```python
from build123d import *

# Parameters (mm, degrees)
SKETCH41_W                                    = 104.14
SKETCH41_H                                    = 148.59
SKETCH41_R                                    = 9.525
EXTRUDE16_DEPTH                               = 16.51
SKETCH42_W                                    = 19.05
SKETCH42_H                                    = 19.05
SKETCH42_W_2                                  = 13.97
SKETCH42_W_3                                  = 12.7
SKETCH42_H_2                                  = 15.24
EXTRUDE17_DEPTH                               = 2.54
F_1_4_CLEARANCE_HOLE3_AT_2_COUNT              = 2
F_1_4_CLEARANCE_HOLE3_AT_2_PITCH              = 88.9
F_1_4_CLEARANCE_HOLE3_AT_3_COUNT              = 2
F_1_4_CLEARANCE_HOLE3_AT_3_PITCH              = 49.6966108
PRESS_PIN_HOLES_FOR_MAGNET_BRACKET_P_2_COUNT  = 2
PRESS_PIN_HOLES_FOR_MAGNET_BRACKET_P_2_PITCH  = 88.9
F_3_32_0_09375_DIAMETER_HOLE1_D               = 2.38125
CBORE_FOR_1_4_SOCKET_HEAD_CAP_SCREW1_AT_COUNT = 2
CBORE_FOR_1_4_SOCKET_HEAD_CAP_SCREW1_AT_PITCH = 57.15
F_1_8_0_125_DIAMETER_HOLE1_AT_2_COUNT         = 2
F_1_8_0_125_DIAMETER_HOLE1_AT_2_PITCH         = 69.85
TAPPED_HOLE_FOR_8_32_HELICOIL1_AT_2_COUNT     = 2
TAPPED_HOLE_FOR_8_32_HELICOIL1_AT_2_PITCH     = 83.29041666
CHAMFER1_SIZE                                 = 5.08


with BuildPart() as part:
    # Sketch41 → Extrude16 (new body)
    with BuildSketch(Plane(origin=(0, 0, 0), x_dir=(1, 0, 0), z_dir=(0, 1, 0))):
        with Locations((0, -36.195)):
            Rectangle(SKETCH41_W, SKETCH41_H)
        with Locations(Location((0, -44.45, 0), (0, 0, 270))):  # turned: the seam where the file's is
            Circle(SKETCH41_R, mode=Mode.SUBTRACT)
    extrude(amount=EXTRUDE16_DEPTH)

    # Sketch42 → Extrude17 (add)
    with BuildSketch(Plane.XZ):
        with Locations((-28.575, 100.965)):
            Rectangle(SKETCH42_W, SKETCH42_H)
        with Locations((45.085, -10.795)):
            Rectangle(SKETCH42_W_2, SKETCH42_H)
        with Locations((0, -30.48)):
            Rectangle(SKETCH42_W_3, SKETCH42_H_2)
        with Locations((-45.085, -10.795)):
            Rectangle(SKETCH42_W_2, SKETCH42_H)
        with Locations((28.575, 100.965)):
            Rectangle(SKETCH42_W, SKETCH42_H)
    extrude(amount=EXTRUDE17_DEPTH)

    # Sketch43 → 1/4 Clearance Hole3 (revolve, cut)
    with BuildSketch(Plane(origin=(-44.45, -2.54, -8.255), x_dir=(0, 0, -1), z_dir=(1, 0, 0))):
        Polygon((0, 0), (0, 19.05), (3.9624, 19.05), (3.57124, 18.65884), (3.57124, 0.39116), (3.9624, 0), align=None)
    f_1_4_clearance_hole3 = revolve(axis=Axis((-44.45, -8.89, -8.255), (0, 1, 0)), mode=Mode.SUBTRACT)

    # 1/4 Clearance Hole3 at 2: 1/4 Clearance Hole3 ×2
    with Locations(*[(i * F_1_4_CLEARANCE_HOLE3_AT_2_PITCH, 0, 0) for i in range(1, F_1_4_CLEARANCE_HOLE3_AT_2_COUNT)]):
        add(f_1_4_clearance_hole3, mode=Mode.SUBTRACT)

    # 1/4 Clearance Hole3 at 3: 1/4 Clearance Hole3 ×2
    with Locations(*[Vector(0.894427191, 0, -0.447213595) * (i * F_1_4_CLEARANCE_HOLE3_AT_3_PITCH) for i in range(1, F_1_4_CLEARANCE_HOLE3_AT_3_COUNT)]):
        add(f_1_4_clearance_hole3, mode=Mode.SUBTRACT)

    # Sketch39 → Press Pin holes for Magnet Bracket Pins (revolve, cut)
    with BuildSketch(Plane(origin=(-44.45, -2.54, -16.51), x_dir=(0, 0, -1), z_dir=(1, 0, 0))):
        Polygon((0, 0), (0, 7.303866233), (1.5875, 6.35), (1.5875, 1.524), (1.6002, 1.524), (1.6002, 0.3048), (1.905, 0), align=None)
    press_pin_holes_for_magnet_bracket_pins = revolve(axis=Axis((-44.45, -8.89, -16.51), (0, 1, 0)), mode=Mode.SUBTRACT)

    # Press Pin holes for Magnet Bracket P 2: Press Pin holes for Magnet Bracket Pins ×2
    with Locations(*[(i * PRESS_PIN_HOLES_FOR_MAGNET_BRACKET_P_2_PITCH, 0, 0) for i in range(1, PRESS_PIN_HOLES_FOR_MAGNET_BRACKET_P_2_COUNT)]):
        add(press_pin_holes_for_magnet_bracket_pins, mode=Mode.SUBTRACT)

    # 3/32 (0.09375) Diameter Hole1 (through all)
    with Locations(Plane(origin=(0, 16.51, 0), x_dir=(-1, 0, 0), z_dir=(0, 1, 0))):
        with Locations((44.45, -16.51), (-44.45, -16.51)):
            Hole(F_3_32_0_09375_DIAMETER_HOLE1_D / 2)

    # Sketch7 → CBORE for 1/4 Socket Head Cap Screw1 (revolve, cut)
    with BuildSketch(Plane(origin=(-28.575, 16.51, 97.79), x_dir=(0, 0, 1), z_dir=(1, 0, 0))):
        Polygon((0, 0), (0, 19.050025), (3.9624, 19.050025), (3.57124, 18.658865), (3.57124, 6.35), (5.55625, 6.35), (5.55625, 0), align=None)
    cbore_for_1_4_socket_head_cap_screw1 = revolve(axis=Axis((-28.575, 22.86, 97.79), (0, -1, 0)), mode=Mode.SUBTRACT)

    # CBORE for 1/4 Socket Head Cap Screw1 at: CBORE for 1/4 Socket Head Cap Screw1 ×2
    with Locations(*[(i * CBORE_FOR_1_4_SOCKET_HEAD_CAP_SCREW1_AT_PITCH, 0, 0) for i in range(1, CBORE_FOR_1_4_SOCKET_HEAD_CAP_SCREW1_AT_COUNT)]):
        add(cbore_for_1_4_socket_head_cap_screw1, mode=Mode.SUBTRACT)

    # Sketch45 → 1/8 (0.125) Diameter Hole1 (revolve, cut)
    with BuildSketch(Plane(origin=(-34.925, -2.54, 105.41), x_dir=(0, 0, -1), z_dir=(1, 0, 0))):
        Polygon((0, 0), (0, 19.05), (1.905, 19.05), (1.63195, 18.77695), (1.63195, 0.27305), (1.905, 0), align=None)
    f_1_8_0_125_diameter_hole1 = revolve(axis=Axis((-34.925, -8.89, 105.41), (0, 1, 0)), mode=Mode.SUBTRACT)

    # 1/8 (0.125) Diameter Hole1 at 2: 1/8 (0.125) Diameter Hole1 ×2
    with Locations(*[(i * F_1_8_0_125_DIAMETER_HOLE1_AT_2_PITCH, 0, 0) for i in range(1, F_1_8_0_125_DIAMETER_HOLE1_AT_2_COUNT)]):
        add(f_1_8_0_125_diameter_hole1, mode=Mode.SUBTRACT)

    # Sketch37 → Tapped Hole for #8-32 Helicoil1 (revolve, cut)
    with BuildSketch(Plane(origin=(-41.64520833, 16.51, 97.79), x_dir=(0, 0, 1), z_dir=(1, 0, 0))):
        Polygon((0, 0), (0, 19.050025), (2.1971, 19.050025), (2.1971, 13.0048), (2.63779, 13.0048), (2.63779, 0.635), (3.27279, 0), align=None)
    tapped_hole_for_8_32_helicoil1 = revolve(axis=Axis((-41.64520833, 22.86, 97.79), (0, -1, 0)), mode=Mode.SUBTRACT)

    # Tapped Hole for #8-32 Helicoil1 at 2: Tapped Hole for #8-32 Helicoil1 ×2
    with Locations(*[(i * TAPPED_HOLE_FOR_8_32_HELICOIL1_AT_2_PITCH, 0, 0) for i in range(1, TAPPED_HOLE_FOR_8_32_HELICOIL1_AT_2_COUNT)]):
        add(tapped_hole_for_8_32_helicoil1, mode=Mode.SUBTRACT)

    # Chamfer1
    chamfer1_edges = [part.edges().sort_by_distance(p)[0] for p in [
        (52.07, 8.255, 110.49),
        (-52.07, 8.255, 110.49),
        (-52.07, 8.255, -38.1),
        (52.07, 8.255, -38.1),
        (0, 16.51, 34.925),
    ]]
    chamfer(chamfer1_edges, length=CHAMFER1_SIZE)


solid = part.part
```
Check sheet for the modelled part. Datum: model origin and axes. Units: mm. A direction names the side the tool comes from. Coordinates: 2 decimals unless noted, no trailing zeros. Write each loop counter-clockwise with the first axis right and the second up, starting at its lowest first coordinate (ties: lowest second). Pieces come first, ordered by that corner, then holes. Notation, with made-up numbers: M -21.5,79 L 10.5,79 A25 cw 10.5,113 Z; hole C 39,77 d6. An arc over 180 degrees is marked long. Write item = value, one per line. Start each with the question number.
1. Thickness scan on probe 1 along X at (y, z) = (0.5, -8); probe 2 along X at (y, z) = (7.25, -16.51); probe 3 along X at (y, z) = (13.75, 97.79). Record the ranges inside material, lowest first.
2. Mould release check, pull along Z, two halves, no side actions. Record for faces 1 (the cylindrical face through (-40.964, 6.857, -7.481)), 2 (the flat face through (4.14, -2.54, -30.37)), 3 (the flat face through (49.57, 8.14, 107.91)), 4 (the cylindrical face through (-46.037, -1.634, -16.302)): pulls with the +Z half, pulls with the -Z half, needs draft (parallel to the pull), parting line crosses it, or undercut.
3. Sectioned sample at A-A (x = 0). Record the cut outline in (y, z) (3 decimals).
4. Go/stop test with flat-tipped pins: pin 1 (2 mm diameter, centred on y = -1.5, z = -30.5, fed in from +X); pin 2 (1.3 mm diameter, centred on y = -1, z = 98, fed in from -X); pin 3 (4.5 mm diameter, centred on x = 28.575, z = 97.79, fed in from +Y); pin 4 (5 mm diameter, centred on x = -35, z = 41, fed in from -Y). Record where each tip stops, or that it passes through.
5. Sectioned sample at B-B (z = -30.48). Record the cut outline in (x, y).
6. Tool access check on faces 5 (the flat face through (-49.49, 8.14, 107.99)), 6 (the cylindrical face through (-42.9, 1.36, -16.17)). Record the directions out of +Z, -Z, +X, -X, +Y, -Y that give a thin tool (end or side, any length) a straight path to the whole face; none if there is none.
7. Sectioned sample at D-D (z = 97.79). State how many separate pieces and enclosed holes the cut face has, then the cut area to 3 significant figures.
8. Sectioned sample at C-C (z = 44.45). Record the cut outline in (x, y) (3 decimals), then the cut area to 3 significant figures.
The answers:
q1.probe_1 = -52.07 to -48.01, -40.89 to 40.89, 48.01 to 52.07
q1.probe_2 = -52.07 to -45.64, -43.26 to 43.26, 45.64 to 52.07
q1.probe_3 = -52.07 to -44.28, -39.01 to -34.13, -23.02 to 23.02, 34.13 to 39.01, 44.28 to 52.07
q2.face_1 = undercut
q2.face_2 = needs draft
q2.face_3 = pulls with the +Z half
q2.face_4 = undercut
q3.outline = M -2.54,-38.1 L 16.51,-38.1 L 16.51,-34.442 L 16.119,-34.051 L -2.149,-34.051 L -2.54,-34.442 Z; M -2.54,-26.518 L -2.149,-26.909 L 16.119,-26.909 L 16.51,-26.518 L 16.51,29.845 L 11.43,34.925 L 0,34.925 L 0,-22.86 L -2.54,-22.86 Z; M 0,53.975 L 11.43,53.975 L 16.51,59.055 L 16.51,110.49 L 0,110.49 Z
q4.pin_1 = 6.35
q4.pin_2 = -38.1
q4.pin_3 = through
q4.pin_4 = 0
q5.outline = M -52.07,0 L -6.35,0 L -6.35,-2.54 L -3.96,-2.54 L -3.57,-2.15 L -3.57,16.12 L -3.96,16.51 L -52.07,16.51 Z; M 3.57,-2.15 L 3.96,-2.54 L 6.35,-2.54 L 6.35,0 L 52.07,0 L 52.07,16.51 L 3.96,16.51 L 3.57,16.12 Z
q6.face_5 = +Z, -X, +Y, -Y
q6.face_6 = -Y
q7.separate_pieces = 5
q7.enclosed_holes = 0
q7.area = 1,320 mm²
q8.outline = M -52.07,0 L -9.525,0 L -9.525,11.43 L -14.605,16.51 L -52.07,16.51 Z; M 9.525,0 L 52.07,0 L 52.07,16.51 L 14.605,16.51 L 9.525,11.43 Z
q8.area = 1,380 mm²
